from build123d import *

# Parameters (mm, degrees)
SKETCH_1_W      = 90
SKETCH_1_H      = 156
EXTRUDE_1_DEPTH = 192
CHAMFER_1_SIZE  = 10
FILLET_1_R      = 4


with BuildPart() as part:
    # 草图1 → 凸台-拉伸1 (new body)
    with BuildSketch(Plane.XY):
        with Locations((45, -78)):
            Rectangle(SKETCH_1_W, SKETCH_1_H)
    extrude(amount=EXTRUDE_1_DEPTH)

    # 倒角1
    chamfer_1_edges = [part.edges().sort_by_distance(p)[0] for p in [
        (0, 0, 96),
        (90, 0, 96),
        (90, -156, 96),
        (0, -156, 96),
    ]]
    chamfer(chamfer_1_edges, length=CHAMFER_1_SIZE)

    # 圆角1
    fillet_1_edges = [part.edges().sort_by_distance(p)[0] for p in [
        (80, -156, 96),
        (10, -156, 96),
        (0, -10, 96),
        (0, -146, 96),
        (90, -10, 96),
        (90, -146, 96),
        (80, 0, 96),
        (10, 0, 96),
    ]]
    fillet(fillet_1_edges, radius=FILLET_1_R)


solid = part.part
Input: part model. Units: mm. Frame: model coordinates. Give positions to 0.01 mm unless a question says otherwise; leave off trailing zeros. Use CSV: the item, a comma, the result in double quotes. Start each with the question number.
Item 1: Line query: line 1 (Y direction, x = 82, z = 131); line 2 (Y direction, x = 81, z = 129). Output: solid intervals per line, ascending.
Item 2: Contact query for a flat-ended pin moving along its axis: P1, Ø2, axis at x = 68.5, y = -92, coming from the -Z side. Output: stop coordinate, or through.
Item 3: Mould query, pull axis Y, two halves, no side actions, for faces 1 (the flat face through (85, -151, 95)), 2 (the flat face through (85, -5, 95)), 3 (the flat face through (44, -77, 0)). Classes: pulls with the +Y half, pulls with the -Y half, needs draft (parallel to the pull), parting line crosses it, or undercut.
Ans:
1,line 1,"y = -154 to -2"
1,line 2,"y = -154.99 to -1.01"
2,P1,"stops at z = 0"
3,face 1,"pulls with the -Y half"
3,face 2,"pulls with the +Y half"
3,face 3,"needs draft"
